```python
from build123d import *

# Parameters (mm, degrees)
SKETCH_W      = 35.56
SKETCH_H      = 17.78
PAD_DEPTH     = 1.6
FILLET_R      = 1
SKETCH001_W   = 5.08
SKETCH001_H   = 4
SKETCH001_W_2 = 3
SKETCH001_H_2 = 5
PAD001_DEPTH  = 2


with BuildPart() as part:
    # Sketch → Pad (new body)
    with BuildSketch(Plane.XY):
        with Locations((17.78, 0)):
            Rectangle(SKETCH_W, SKETCH_H)
    extrude(amount=PAD_DEPTH)

    # Fillet
    fillet_edges = [part.edges().sort_by_distance(p)[0] for p in [
        (0, -8.89, 0.8),
        (0, 8.89, 0.8),
        (35.56, -8.89, 0.8),
        (35.56, 8.89, 0.8),
    ]]
    fillet(fillet_edges, radius=FILLET_R)

    # Sketch001 (on Face5 of Fillet) → Pad001 (join)
    with BuildSketch(Plane.XY.offset(1.6)):
        with Locations((2.54, 0)):
            Rectangle(SKETCH001_W, SKETCH001_H)
        with Locations((30.5, 0)):
            Rectangle(SKETCH001_W_2, SKETCH001_H_2)
    extrude(amount=PAD001_DEPTH)


solid = part.part
```
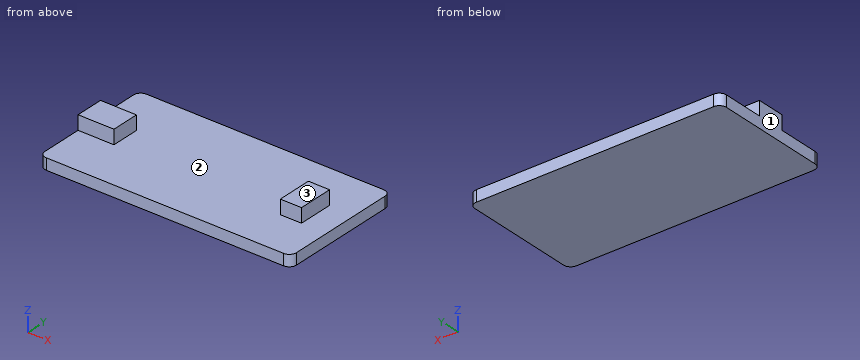
Model file for the job. Use its own axes, mm. Face numbers are marked on the shaded views. Coordinates: 2 decimals unless noted, no trailing zeros. Loops run counter-clockwise (first coordinate to the right, second up) from the corner with the lowest first, then second, coordinate; pieces in that order, holes last. Notation, with made-up numbers: (-23.5, 50) - (21.5, 50) arc R18 cw to (21.5, 69) - close; hole circle Ø2 at (63.25, 85.25). An arc over 180 degrees is marked (long way). Answer as a JSON object with one key per item and string values. Group by question number.
(1) Cut at A-A (z = 2.65). Give the cut face in (x, y), then the cut area to 3 significant figures.
(2) Probe line 1 along X through (y, z) = (-0.5, 2.25); line 2 along Z through (x, y) = (18, -7); line 3 along X through (y, z) = (-8, 1.35). List the from-to ranges inside material, lowest first.
(3) Cut at D-D (y = 3.75). Give the cut face in (x, z), then the cut area to 3 significant figures.
(4) Cut at C-C (x = 2.5). Give the cut face in (y, z), then the cut area to 3 significant figures.
(5) Cut at B-B (y = -1.25). Give the cut face in (x, z), then the cut area to 3 significant figures.
(6) Two-plate mould, pull along X, no slides. Class the marked faces 1, 2 and 3: released by +X, released by -X, zero draft, split by the parting line, or undercut.
(7) Flat gauge pins, fed straight in: pin 1 (1 mm diameter, centred on y = 1, z = 2.5, fed in from +X); pin 2 (0.6 mm diameter, centred on x = 30.5, z = 2.5, fed in from -Y); pin 3 (1 mm diameter, centred on x = 2.5, z = 3, fed in from +Y). Where does each tip first touch, or does it go through?
Geometry says:
{
 "1": {"outline": "(0, -2) - (5.08, -2) - (5.08, 2) - (0, 2) - close; (29, -2.5) - (32, -2.5) - (32, 2.5) - (29, 2.5) - close", "area": "35.3 mm^2"},
 "2": {"line 1": "x = 0 to 5.08, 29 to 32", "line 2": "z = 0 to 1.6", "line 3": "x = 0.01 to 35.55"},
 "3": {"outline": "(0, 0) - (35.56, 0) - (35.56, 1.6) - (0, 1.6) - close", "area": "56.9 mm^2"},
 "4": {"outline": "(-8.89, 0) - (8.89, 0) - (8.89, 1.6) - (2, 1.6) - (2, 3.6) - (-2, 3.6) - (-2, 1.6) - (-8.89, 1.6) - close", "area": "36.4 mm^2"},
 "5": {"outline": "(0, 0) - (35.56, 0) - (35.56, 1.6) - (32, 1.6) - (32, 3.6) - (29, 3.6) - (29, 1.6) - (5.08, 1.6) - (5.08, 3.6) - (0, 3.6) - close", "area": "73.1 mm^2"},
 "6": {"face 1": "released by -X", "face 2": "undercut", "face 3": "zero draft"},
 "7": {"pin 1": "stops at x = 32", "pin 2": "stops at y = -2.5", "pin 3": "stops at y = 2"}
}
